Source: CAD feature listing. Evaluate the final solid. Frame: model axes, mm. Face numbers are marked on the shaded views. A direction names the side the tool comes from. Coordinates: 2 decimals unless noted, no trailing zeros. Write each loop counter-clockwise with the first axis right and the second up, starting at its lowest first coordinate (ties: lowest second). Pieces come first, ordered by that corner, then holes. Notation, with made-up numbers: (-29.5, -27.5) -> (-5.5, -27.5) arc R18 ccw to (-5.5, -5.5) -> close; hole circle Ø2 at (51, -40). An arc over 180 degrees is marked (long way). Write item = value, one per line.
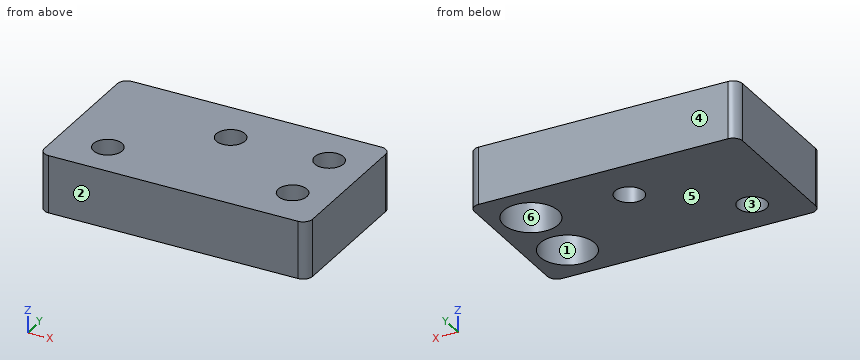
from build123d import *

# Parameters (mm, degrees)
SKETCH_1_W          = 28
SKETCH_1_H          = 16
EXTRUDE_1_DEPTH     = 6
SKETCH_2_R          = 2.85
CUT_EXTRUDE_1_DEPTH = 3.2
SKETCH_3_R          = 1.5
CUT_EXTRUDE_2_DEPTH = 3.2
FILLET_1_R          = 1
SKETCH_4_R          = 1.5
CUT_EXTRUDE_3_DEPTH = 10


with BuildPart() as part:
    # 草图1 → 凸台-拉伸1 (new body)
    with BuildSketch(Plane.XY):
        Rectangle(SKETCH_1_W, SKETCH_1_H)
    extrude(amount=EXTRUDE_1_DEPTH)

    # 草图2 → 切除-拉伸1 (cut)
    with BuildSketch(Plane(origin=(0, 0, 0), x_dir=(-1, 0, 0), z_dir=(0, 0, -1))):
        with Locations((-10, 3.5)):
            Circle(SKETCH_2_R)
        with Locations((-10, -3.5)):
            Circle(SKETCH_2_R)
    extrude(amount=-CUT_EXTRUDE_1_DEPTH, mode=Mode.SUBTRACT)

    # 草图3 → 切除-拉伸2 (cut)
    with BuildSketch(Plane(origin=(0, 0, 3.2), x_dir=(-1, 0, 0), z_dir=(0, 0, -1))):
        with Locations((-10, 3.5)):
            Circle(SKETCH_3_R)
        with Locations((-10, -3.5)):
            Circle(SKETCH_3_R)
    extrude(amount=-CUT_EXTRUDE_2_DEPTH, mode=Mode.SUBTRACT)

    # 圆角1
    fillet_1_edges = [part.edges().sort_by_distance(p)[0] for p in [
        (-14, 8, 3),
        (14, 8, 3),
        (14, -8, 3),
        (-14, -8, 3),
    ]]
    fillet(fillet_1_edges, radius=FILLET_1_R)

    # 草图4 → 切除-拉伸3 (cut)
    with BuildSketch(Plane.XY.offset(6)):
        with Locations((0, 3)):
            Circle(SKETCH_4_R)
        with Locations((-9, -4)):
            Circle(SKETCH_4_R)
    extrude(amount=-CUT_EXTRUDE_3_DEPTH, mode=Mode.SUBTRACT)


solid = part.part
1) Reachability of the marked faces 1 and 2 from +Z, -Z, +X, -X, +Y, -Y: full face, straight path, thin tool, end or side. Return the list, or none.
Answer block:
face_1 = -Z
face_2 = +Z, -Z, +X, -X, -Y
2) Cut plane B-B, the plane x = 0. Output: boundary loops of the cut face in (y, z), and give its area (3 significant figures).
Answer block:
outline = (-8, 0) -> (1.5, 0) -> (1.5, 6) -> (-8, 6) -> close; (4.5, 0) -> (8, 0) -> (8, 6) -> (4.5, 6) -> close
area = 78.0 mm2
3) Pull-direction query (Y, two-part tool) for the marked faces 3, 4, 5 and 6; classes: +Y half, -Y half, draft (parallel to the pull), parting line (faces both ways), or undercut.
Answer block:
face_3 = undercut
face_4 = +Y half
face_5 = draft
face_6 = undercut
4) Cut plane D-D, the plane z = 0.85. Output: boundary loops of the cut face in (x, y).
Answer block:
outline = (-14, -7) arc R1 ccw to (-13, -8) -> (13, -8) arc R1 ccw to (14, -7) -> (14, 7) arc R1 ccw to (13, 8) -> (-13, 8) arc R1 ccw to (-14, 7) -> close; hole circle Ø3 at (-9, -4); hole circle Ø3 at (0, 3); hole circle Ø5.7 at (10, -3.5); hole circle Ø5.7 at (10, 3.5)
5) First-contact query: pin 1 Ø3.5 at (x, y) = (10, -3.5) entering from +Z; pin 2 Ø5 at (x, y) = (10, 3.5) entering from -Z; pin 3 Ø1.7 at (x, y) = (10.5, -3.5) entering from -Z. Flat tips, straight axial feed; report the tip coordinate or a pass-through.
Answer block:
pin_1 = 6
pin_2 = 3.2
pin_3 = through
6) Material intervals for probe 1 along Y at (x, z) = (10, 3.8); probe 2 along Y at (x, z) = (10, 2.3); probe 3 along Y at (x, z) = (0, 4.2), sorted ascending. Write a range as [from, to].
Answer block:
probe_1 = [-8, -5], [-2, 2], [5, 8]
probe_2 = [-8, -6.35], [-0.65, 0.65], [6.35, 8]
probe_3 = [-8, 1.5], [4.5, 8]
7) Cut plane C-C, the plane y = 3.5. Output: boundary loops of the cut face in (x, z).
Answer block:
outline = (-14, 0) -> (-1.41, 0) -> (-1.41, 6) -> (-14, 6) -> close; (1.41, 0) -> (7.15, 0) -> (7.15, 3.2) -> (8.5, 3.2) -> (8.5, 6) -> (1.41, 6) -> close; (11.5, 3.2) -> (12.85, 3.2) -> (12.85, 0) -> (14, 0) -> (14, 6) -> (11.5, 6) -> close
8) Cut plane A-A, the plane x = 10. Output: boundary loops of the cut face in (y, z), and give its area (3 significant figures).
Answer block:
outline = (-8, 0) -> (-6.35, 0) -> (-6.35, 3.2) -> (-5, 3.2) -> (-5, 6) -> (-8, 6) -> close; (-2, 3.2) -> (-0.65, 3.2) -> (-0.65, 0) -> (0.65, 0) -> (0.65, 3.2) -> (2, 3.2) -> (2, 6) -> (-2, 6) -> close; (5, 3.2) -> (6.35, 3.2) -> (6.35, 0) -> (8, 0) -> (8, 6) -> (5, 6) -> close
area = 42.7 mm2
